Geometry: see drawing. Coordinates: mm, zero at the bounding-box minimum. Give positions to 0.01 mm unless a question says otherwise; leave off trailing zeros. Loops run counter-clockwise (first coordinate to the right, second up) from the corner with the lowest first, then second, coordinate; pieces in that order, holes last. Notation, with made-up numbers: M -11,50.5 L 19,50.5 A13 cw 19,72.5 Z; hole C -11.5,24.5 d3. An arc over 180 degrees is marked long. Answer in a Markdown table with one row per item.
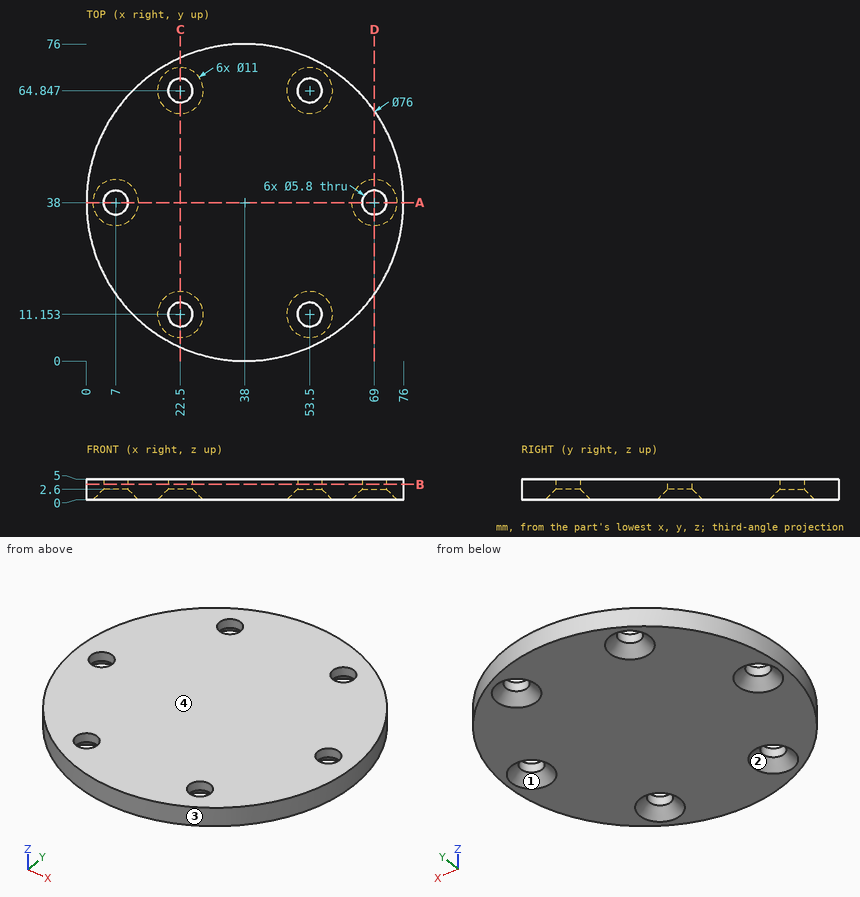
1) Section A-A, the plane y = 38. Return loops of the section in (x, z).
Reply:
| item | result |
|---|---|
| outline | M 0,0 L 1.5,0 L 4.1,2.6 L 4.1,5 L 0,5 Z; M 9.9,2.6 L 12.5,0 L 63.5,0 L 66.1,2.6 L 66.1,5 L 9.9,5 Z; M 71.9,2.6 L 74.5,0 L 76,0 L 76,5 L 71.9,5 Z |
2) Section C-C, the plane x = 22.5. Return loops of the section in (y, z) (1 decimal), then the cut area to 3 significant figures.
Reply:
| item | result |
|---|---|
| outline | M 3.3,0 L 5.7,0 L 8.3,2.6 L 8.3,5 L 3.3,5 Z; M 14.1,2.6 L 16.7,0 L 59.3,0 L 61.9,2.6 L 61.9,5 L 14.1,5 Z; M 67.7,2.6 L 70.3,0 L 72.7,0 L 72.7,5 L 67.7,5 Z |
| area | 275 mm² |
3) Section B-B, the plane z = 3.7. Return loops of the section in (x, y), then the cut area to 3 significant figures.
Reply:
| item | result |
|---|---|
| outline | C 38,38 d76; hole C 7,38 d5.8; hole C 22.5,11.15 d5.8; hole C 22.5,64.85 d5.8; hole C 53.5,11.15 d5.8; hole C 53.5,64.85 d5.8; hole C 69,38 d5.8 |
| area | 4,380 mm² |
4) Pull-direction query (X, two-part tool) for the marked faces 1, 2, 3 and 4; classes: released by +X, released by -X, zero draft, split by the parting line, or undercut.
Reply:
| item | result |
|---|---|
| face 1 | undercut |
| face 2 | undercut |
| face 3 | split by the parting line |
| face 4 | zero draft |
5) Section D-D, the plane x = 69. Return loops of the section in (y, z).
Reply:
| item | result |
|---|---|
| outline | M 16.02,0 L 32.5,0 L 35.1,2.6 L 35.1,5 L 16.02,5 Z; M 40.9,2.6 L 43.5,0 L 59.98,0 L 59.98,5 L 40.9,5 Z |
6) Pin query (flat end, axial travel): pin 1 Ø4.5 at (x, y) = (69, 38) entering from +Z; pin 2 Ø2 at (x, z) = (66.5, 0.5) entering from -Y (1 decimal); pin 3 Ø1.5 at (y, z) = (48, 4.5) entering from +X; pin 4 Ø3 at (x, z) = (67.5, 2.5) entering from +Y. Return the tip coordinate at first contact, or that it passes through.
Reply:
| item | result |
|---|---|
| pin 1 | passes through |
| pin 2 | stops at y = 11.8 |
| pin 3 | stops at x = 74.86 |
| pin 4 | stops at y = 63.69 |
7) Material intervals for L1, parallel to Y at x = 22, z = 3.35; L2, parallel to Y at x = 53, z = 2.95; L3, parallel to Y at x = 9.5, z = 3.85 (1 decimal), sorted ascending.
Reply:
| item | result |
|---|---|
| L1 | y = 3.53 to 8.3, 14.01 to 61.99, 67.7 to 72.47 |
| L2 | y = 3.09 to 8.3, 14.01 to 61.99, 67.7 to 72.91 |
| L3 | y = 12.9 to 36.5, 39.5 to 63.1 |
